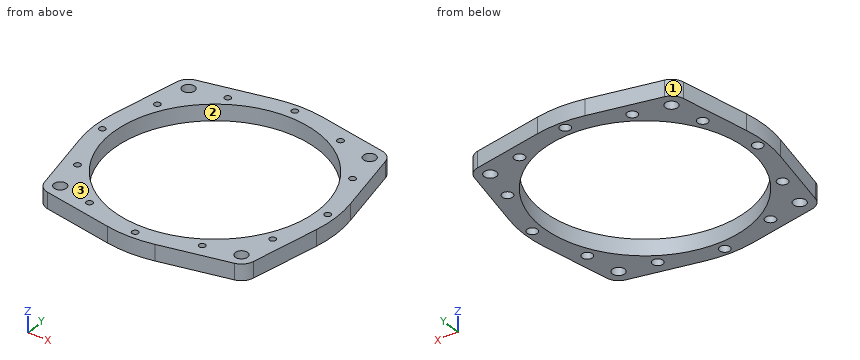
```python
from build123d import *

# Parameters (mm, degrees)
SKETCH_1_R          = 3.1
SKETCH_1_R_2        = 1.6
SKETCH_1_R_3        = 51
EXTRUDE_1_DEPTH     = 8
SKETCH_2_R          = 2.6
CUT_EXTRUDE_1_DEPTH = 4


with BuildPart() as part:
    # 草图1 → 凸台-拉伸1 (new body)
    with BuildSketch(Plane.XY):
        with BuildLine():
            Line((-51.862164548, 46.382279896), (-58.818553272, 11.848113395))
            ThreePointArc((-58.818553272, 11.848113395), (-60, 0), (-58.818553272, -11.848113395))
            Line((-58.818553272, -11.848113395), (-51.862164548, -46.382279896))
            ThreePointArc((-51.862164548, -46.382279896), (-49.949747468, -49.949747468), (-46.382279896, -51.862164548))
            Line((-46.382279896, -51.862164548), (-11.848113395, -58.818553272))
            ThreePointArc((-11.848113395, -58.818553272), (0, -60), (11.848113395, -58.818553272))
            Line((11.848113395, -58.818553272), (46.382279896, -51.862164548))
            ThreePointArc((46.382279896, -51.862164548), (49.949747468, -49.949747468), (51.862164548, -46.382279896))
            Line((51.862164548, -46.382279896), (58.818553272, -11.848113395))
            ThreePointArc((58.818553272, -11.848113395), (60, 0), (58.818553272, 11.848113395))
            Line((58.818553272, 11.848113395), (51.862164548, 46.382279896))
            ThreePointArc((51.862164548, 46.382279896), (49.949747468, 49.949747468), (46.382279896, 51.862164548))
            Line((46.382279896, 51.862164548), (11.848113395, 58.818553272))
            ThreePointArc((11.848113395, 58.818553272), (0, 60), (-11.848113395, 58.818553272))
            Line((-11.848113395, 58.818553272), (-46.382279896, 51.862164548))
            ThreePointArc((-46.382279896, 51.862164548), (-49.949747468, 49.949747468), (-51.862164548, 46.382279896))
        make_face()
        with Locations((45, 45)):
            Circle(SKETCH_1_R, mode=Mode.SUBTRACT)
        with Locations((-45, 45)):
            Circle(SKETCH_1_R, mode=Mode.SUBTRACT)
        with Locations((-45, -45)):
            Circle(SKETCH_1_R, mode=Mode.SUBTRACT)
        with Locations((45, -45)):
            Circle(SKETCH_1_R, mode=Mode.SUBTRACT)
        with Locations((0, 56)):
            Circle(SKETCH_1_R_2, mode=Mode.SUBTRACT)
        with Locations((28, 48.497422612)):
            Circle(SKETCH_1_R_2, mode=Mode.SUBTRACT)
        with Locations((48.497422612, 28)):
            Circle(SKETCH_1_R_2, mode=Mode.SUBTRACT)
        with Locations((56, 0)):
            Circle(SKETCH_1_R_2, mode=Mode.SUBTRACT)
        with Locations((48.497422612, -28)):
            Circle(SKETCH_1_R_2, mode=Mode.SUBTRACT)
        with Locations((28, -48.497422612)):
            Circle(SKETCH_1_R_2, mode=Mode.SUBTRACT)
        with Locations((0, -56)):
            Circle(SKETCH_1_R_2, mode=Mode.SUBTRACT)
        with Locations((-28, -48.497422612)):
            Circle(SKETCH_1_R_2, mode=Mode.SUBTRACT)
        with Locations((-48.497422612, -28)):
            Circle(SKETCH_1_R_2, mode=Mode.SUBTRACT)
        with Locations((-56, 0)):
            Circle(SKETCH_1_R_2, mode=Mode.SUBTRACT)
        with Locations((-48.497422612, 28)):
            Circle(SKETCH_1_R_2, mode=Mode.SUBTRACT)
        with Locations((-28, 48.497422612)):
            Circle(SKETCH_1_R_2, mode=Mode.SUBTRACT)
        Circle(SKETCH_1_R_3, mode=Mode.SUBTRACT)
    extrude(amount=EXTRUDE_1_DEPTH)

    # 草图2 → 切除-拉伸1 (cut)
    with BuildSketch(Plane(origin=(0, 0, 0), x_dir=(-1, 0, 0), z_dir=(0, 0, -1))):
        with Locations((-28, 48.497422612)):
            Circle(SKETCH_2_R)
        with Locations((0, 56)):
            Circle(SKETCH_2_R)
        with Locations((28, 48.497422612)):
            Circle(SKETCH_2_R)
        with Locations((48.497422612, 28)):
            Circle(SKETCH_2_R)
        with Locations((56, 0)):
            Circle(SKETCH_2_R)
        with Locations((48.497422612, -28)):
            Circle(SKETCH_2_R)
        with Locations((28, -48.497422612)):
            Circle(SKETCH_2_R)
        with Locations((0, -56)):
            Circle(SKETCH_2_R)
        with Locations((-28, -48.497422612)):
            Circle(SKETCH_2_R)
        with Locations((-48.497422612, -28)):
            Circle(SKETCH_2_R)
        with Locations((-56, 0)):
            Circle(SKETCH_2_R)
        with Locations((-48.497422612, 28)):
            Circle(SKETCH_2_R)
    extrude(amount=-CUT_EXTRUDE_1_DEPTH, mode=Mode.SUBTRACT)


solid = part.part
```
Input: part model. Units: mm. Frame: model coordinates. Face numbers are marked on the shaded views. Round coordinates to 2 decimals unless told otherwise and drop trailing zeros. Loops run counter-clockwise (first coordinate to the right, second up) from the corner with the lowest first, then second, coordinate; pieces in that order, holes last. Notation, with made-up numbers: M 43,88.5 L 53,88.5 A17 cw 53,111.5 Z; hole C 51,8.25 d9. An arc over 180 degrees is marked long. Answer in a Markdown table with one row per item. Add a question column.
1. Contact query for flat-ended pins moving along their axis: pin 1 (4 mm diameter, centred on y = 9.5, z = 4, fed in from +X); pin 2 (2.5 mm diameter, centred on x = -28.5, y = -49.5, fed in from -Z); pin 3 (1.5 mm diameter, centred on x = 46.5, z = 2.5, fed in from +Y). Output: stop coordinate, or through.
2. Section D-D (y = -56). Output: boundary loops of the cut face in (x, z), and give its area (3 significant figures).
3. Ray query, probe 1 along Y at (x, z) = (28, 1.2) (3 decimals); probe 2 along Y at (x, z) = (20, 7.75); probe 3 along Y at (x, z) = (-38, 0.75). Return the intervals inside material, ascending.
4. Section C-C (x = -38). Output: boundary loops of the cut face in (y, z), and give its area (3 significant figures).
5. Section B-B (y = 22). Output: boundary loops of the cut face in (x, z).
6. Section A-A (x = 0). Output: boundary loops of the cut face in (y, z), and give its area (3 significant figures).
7. Mould query, pull axis X, two halves, no side actions, for the marked faces 1, 2 and 3. Classes: released by +X, released by -X, zero draft, split by the parting line, or undercut.
Values follow:
| question | item | result |
|---|---|---|
| 1 | pin 1 | x = 59.53 |
| 1 | pin 2 | z = 4 |
| 1 | pin 3 | y = 51.99 |
| 2 | outline | M -25.84,0 L -2.6,0 L -2.6,4 L -1.6,4 L -1.6,8 L -25.84,8 Z; M 1.6,4 L 2.6,4 L 2.6,0 L 25.84,0 L 25.84,8 L 1.6,8 Z |
| 2 | area | 380 mm^2 |
| 3 | probe 1 | -55.565 to -51.097, -45.897 to -42.626, 42.626 to 45.897, 51.097 to 55.565 |
| 3 | probe 2 | -57.18 to -46.91, 46.91 to 57.18 |
| 3 | probe 3 | -53.55 to -34.01, 34.01 to 53.55 |
| 4 | outline | M -53.55,0 L -34.01,0 L -34.01,8 L -53.55,8 Z; M 34.01,0 L 53.55,0 L 53.55,8 L 34.01,8 Z |
| 4 | area | 313 mm^2 |
| 5 | outline | M -56.77,0 L -46.01,0 L -46.01,8 L -56.77,8 Z; M 46.01,0 L 56.77,0 L 56.77,8 L 46.01,8 Z |
| 6 | outline | M -60,0 L -58.6,0 L -58.6,4 L -57.6,4 L -57.6,8 L -60,8 Z; M -54.4,4 L -53.4,4 L -53.4,0 L -51,0 L -51,8 L -54.4,8 Z; M 51,0 L 53.4,0 L 53.4,4 L 54.4,4 L 54.4,8 L 51,8 Z; M 57.6,4 L 58.6,4 L 58.6,0 L 60,0 L 60,8 L 57.6,8 Z |
| 6 | area | 76.8 mm^2 |
| 7 | face 1 | released by -X |
| 7 | face 2 | undercut |
| 7 | face 3 | zero draft |
